```python
from build123d import *

# Parameters (mm, degrees)
SKETCH1_W           = 26
SKETCH1_H           = 11
BOSS_EXTRUDE1_DEPTH = 1.8
FILLET1_R           = 0.2
SKETCH2_R           = 1
CUT_EXTRUDE1_DEPTH  = 153.699256387
FILLET2_R           = 0.5
FILLET3_R           = 0.2
SKETCH4_W           = 12.5
SKETCH4_H           = 1
BOSS_EXTRUDE2_DEPTH = 3.7
FILLET4_R           = 0.25
FILLET5_R           = 0.25


with BuildPart() as part:
    # Sketch1 → Boss-Extrude1 (new body)
    with BuildSketch(Plane.XY.offset(13.74095281)):
        with Locations((74.443158301, -119.669952335)):
            Rectangle(SKETCH1_W, SKETCH1_H)
    extrude(amount=-BOSS_EXTRUDE1_DEPTH)

    # Fillet1
    fillet1_edges = [part.edges().sort_by_distance(p)[0] for p in [
        (87.443158301, -119.669952335, 13.74095281),
        (74.443158301, -114.169952335, 13.74095281),
        (61.443158301, -119.669952335, 13.74095281),
        (74.443158301, -125.169952335, 13.74095281),
    ]]
    fillet(fillet1_edges, radius=FILLET1_R)

    # Sketch2 → Cut-Extrude1 (cut, through all)
    with BuildSketch(Plane.XY.offset(13.74095281)):
        with Locations((84.443158301, -122.169952335)):
            Circle(SKETCH2_R)
    extrude(amount=-CUT_EXTRUDE1_DEPTH, mode=Mode.SUBTRACT)

    # Fillet2
    # the kernel refuses this fillet: 0.5 mm, written as the material it takes off along each edge
    with BuildSketch(Plane(origin=(86.943158301, -124.669952335, 13.74095281), x_dir=(0, -1, 0), z_dir=(-1, 0, 0))) as fillet2_piece_1:
        with BuildLine():
            CenterArc((0.3, -0.2), 0.2, 0, 90)
            Line((0.5, -0.2), (0.5, 0))
            Line((0.5, 0), (0.3, 0))
        make_face()
    revolve(axis=Axis((86.943158301, -124.669952335, 13.74095281), (0, 0, 1)), revolution_arc=90, mode=Mode.SUBTRACT)
    with BuildSketch(Plane(origin=(61.943158301, -124.669952335, 13.74095281), x_dir=(-1, 0, 0), z_dir=(0, 1, 0))) as fillet2_piece_2:
        with BuildLine():
            CenterArc((0.3, -0.2), 0.2, 0, 90)
            Line((0.5, -0.2), (0.5, 0))
            Line((0.5, 0), (0.3, 0))
        make_face()
    revolve(axis=Axis((61.943158301, -124.669952335, 13.74095281), (0, 0, 1)), revolution_arc=90, mode=Mode.SUBTRACT)
    with BuildSketch(Plane(origin=(86.943158301, -114.669952335, 13.74095281), x_dir=(1, 0, 0), z_dir=(0, -1, 0))) as fillet2_piece_3:
        with BuildLine():
            CenterArc((0.3, -0.2), 0.2, 0, 90)
            Line((0.5, -0.2), (0.5, 0))
            Line((0.5, 0), (0.3, 0))
        make_face()
    revolve(axis=Axis((86.943158301, -114.669952335, 13.74095281), (0, 0, 1)), revolution_arc=90, mode=Mode.SUBTRACT)
    with BuildSketch(Plane(origin=(61.943158301, -114.669952335, 13.74095281), x_dir=(0, 1, 0), z_dir=(1, 0, 0))) as fillet2_piece_4:
        with BuildLine():
            CenterArc((0.3, -0.2), 0.2, 0, 90)
            Line((0.5, -0.2), (0.5, 0))
            Line((0.5, 0), (0.3, 0))
        make_face()
    revolve(axis=Axis((61.943158301, -114.669952335, 13.74095281), (0, 0, 1)), revolution_arc=90, mode=Mode.SUBTRACT)
    with BuildSketch(Plane(origin=(87.443158301, -125.169952335, 13.74095281), x_dir=(-1, 0, 0), z_dir=(0, 0, -1)), Plane(origin=(87.443158301, -114.169952335, 13.74095281), x_dir=(0, -1, 0), z_dir=(0, 0, -1))) as fillet2_piece_5:
        with BuildLine():
            CenterArc((FILLET2_R, FILLET2_R), FILLET2_R, 180, 90)
            Line((0, FILLET2_R), (0, 0))
            Line((0, 0), (FILLET2_R, 0))
        make_face()
    extrude(amount=3.05, mode=Mode.SUBTRACT)
    with BuildSketch(Plane(origin=(61.443158301, -114.169952335, 13.74095281), x_dir=(0, -1, 0), z_dir=(0, 0, -1)), Plane(origin=(61.443158301, -125.169952335, 13.74095281), x_dir=(1, 0, 0), z_dir=(0, 0, -1))) as fillet2_piece_6:
        with BuildLine():
            CenterArc((FILLET2_R, -FILLET2_R), FILLET2_R, 90, 90)
            Line((0, -FILLET2_R), (0, 0))
            Line((0, 0), (FILLET2_R, 0))
        make_face()
    extrude(amount=3.05, mode=Mode.SUBTRACT)

    # Fillet3
    fillet3_edges = [part.edges().sort_by_distance(p)[0] for p in [
        (83.443158301, -122.169952335, 11.94095281),
        (83.443158301, -122.169952335, 13.74095281),
    ]]
    fillet(fillet3_edges, radius=FILLET3_R)

    # Sketch4 → Boss-Extrude2 (add)
    with BuildSketch(Plane(origin=(0, 0, 11.94095281), x_dir=(-1, 0, 0), z_dir=(0, 0, -1))):
        with Locations((-74.443158301, -124.669952335)):
            Rectangle(SKETCH4_W, SKETCH4_H)
        with Locations((-74.443158301, -114.669952335)):
            Rectangle(SKETCH4_W, SKETCH4_H)
    extrude(amount=BOSS_EXTRUDE2_DEPTH)

    # Fillet4
    fillet4_edges = [part.edges().sort_by_distance(p)[0] for p in [
        (61.443158301, -119.669952335, 11.94095281),
        (65.068158301, -125.169952335, 11.94095281),
        (83.818158301, -114.169952335, 11.94095281),
        (87.443158301, -119.669952335, 11.94095281),
        (87.296711691, -125.023505725, 11.94095281),
        (87.296711691, -114.316398944, 11.94095281),
        (61.58960491, -114.316398944, 11.94095281),
        (61.58960491, -125.023505725, 11.94095281),
        (83.818158301, -125.169952335, 11.94095281),
        (65.068158301, -114.169952335, 11.94095281),
        (74.443158301, -125.169952335, 8.24095281),
        (74.443158301, -124.169952335, 8.24095281),
        (74.443158301, -114.169952335, 8.24095281),
        (74.443158301, -115.169952335, 8.24095281),
    ]]
    fillet(fillet4_edges, radius=FILLET4_R)

    # Fillet5
    fillet5_edges = [part.edges().sort_by_distance(p)[0] for p in [
        (68.193158301, -114.169952335, 10.34095281),
        (68.193158301, -114.243175639, 8.314176115),
        (68.193158301, -115.169952335, 10.21595281),
        (68.193158301, -115.09672903, 8.314176115),
        (68.193158301, -125.169952335, 10.34095281),
        (68.193158301, -125.09672903, 8.314176115),
        (68.193158301, -124.169952335, 10.21595281),
        (68.193158301, -124.243175639, 8.314176115),
        (80.693158301, -125.169952335, 10.34095281),
        (80.693158301, -125.09672903, 8.314176115),
        (80.693158301, -124.169952335, 10.21595281),
        (80.693158301, -124.243175639, 8.314176115),
        (80.693158301, -114.169952335, 10.34095281),
        (80.693158301, -114.243175639, 8.314176115),
        (80.693158301, -115.169952335, 10.21595281),
        (80.693158301, -115.09672903, 8.314176115),
        (68.193158301, -114.669952335, 8.24095281),
        (68.193158301, -124.669952335, 8.24095281),
        (80.693158301, -124.669952335, 8.24095281),
        (80.693158301, -114.669952335, 8.24095281),
    ]]
    fillet(fillet5_edges, radius=FILLET5_R)


solid = part.part
```
Can you work these out from the model? Positions are in its coordinate system, mm. A direction names the side the tool comes from. Give positions to 0.01 mm unless a question says otherwise; leave off trailing zeros. Order: outer loops, then holes, each group sorted by start corner. A loop starts at its lowest first (then second) coordinate and runs counter-clockwise, first axis right, second up. Notation, with made-up numbers: M -10,-30 L 30,-30 A28 ccw 30,-8 Z; hole C 63,-26 d10. An arc over 180 degrees is marked long. Write item = value, one per line. Start each with the question number.
Q1. I need wall thicknesses on probe 1 along Y at (x, z) = (71, 11.4); probe 2 along Z at (x, y) = (69.25, -124); probe 3 along X at (y, z) = (-121.75, 12.35). Which ranges of each line are inside material? Lowest first, please. Write a range as [from, to].
Q2. For faces 4 (the flat face through (74, -125.17, 12)), 5 (the flat face through (75, -115.17, 10)), which set-ups out of +Z, -Z, +X, -X, +Y, -Y let a thin tool reach every point of the face, with its end or its side?
Q3. We'd pull the mould along Y, two halves only. Please class faces 1 (the flat face through (75, -124.17, 10)), 2 (the flat face through (61.443, -120, 13)), 3 (the flat face through (74, -114.17, 12)): pulls with the +Y half, pulls with the -Y half, needs draft (parallel to the pull), parting line crosses it, or undercut.
Q4. Suppose I cut it at B-B (x = 72.25). Write out the boundary of the cut face in (y, z).
Q5. Will these pins go through, and if not, where does the flat tip stop? pin 1 Ø2.5 at (x, y) = (84.44, -122.17) entering from -Z; pin 2 Ø0.6 at (y, z) = (-114.5, 10) entering from +X; pin 3 Ø0.6 at (y, z) = (-114.5, 9.5) entering from -X.
Q6. Suppose I cut it at A-A (z = 9.7). Write out the boundary of the cut face in (x, y), plus the area to 3 significant figures.
Q7. Suppose I cut it at C-C (y = -119.5). Write out the boundary of the cut face in (x, z), plus the area to 3 significant figures.
Check result:
q1.probe_1 = [-125.17, -124.17], [-115.17, -114.17]
q1.probe_2 = [11.94, 13.74]
q1.probe_3 = [61.44, 83.54], [85.35, 87.44]
q2.face_4 = +Z, -Z, +X, -X, -Y
q2.face_5 = -Z, +X, -X
q3.face_1 = undercut
q3.face_2 = needs draft
q3.face_3 = pulls with the +Y half
q4.outline = M -125.17,8.49 A0.25 ccw -124.92,8.24 L -124.42,8.24 A0.25 ccw -124.17,8.49 L -124.17,11.94 L -115.17,11.94 L -115.17,8.49 A0.25 ccw -114.92,8.24 L -114.42,8.24 A0.25 ccw -114.17,8.49 L -114.17,13.54 A0.2 ccw -114.37,13.74 L -124.97,13.74 A0.2 ccw -125.17,13.54 Z
q5.pin_1 = 11.94
q5.pin_2 = 80.69
q5.pin_3 = 68.19
q6.outline = M 68.19,-124.92 A0.25 ccw 68.44,-125.17 L 80.44,-125.17 A0.25 ccw 80.69,-124.92 L 80.69,-124.42 A0.25 ccw 80.44,-124.17 L 68.44,-124.17 A0.25 ccw 68.19,-124.42 Z; M 68.19,-114.92 A0.25 ccw 68.44,-115.17 L 80.44,-115.17 A0.25 ccw 80.69,-114.92 L 80.69,-114.42 A0.25 ccw 80.44,-114.17 L 68.44,-114.17 A0.25 ccw 68.19,-114.42 Z
q6.area = 24.9 mm2
q7.outline = M 61.44,12.19 A0.25 ccw 61.69,11.94 L 87.19,11.94 A0.25 ccw 87.44,12.19 L 87.44,13.54 A0.2 ccw 87.24,13.74 L 61.64,13.74 A0.2 ccw 61.44,13.54 Z
q7.area = 46.8 mm2
